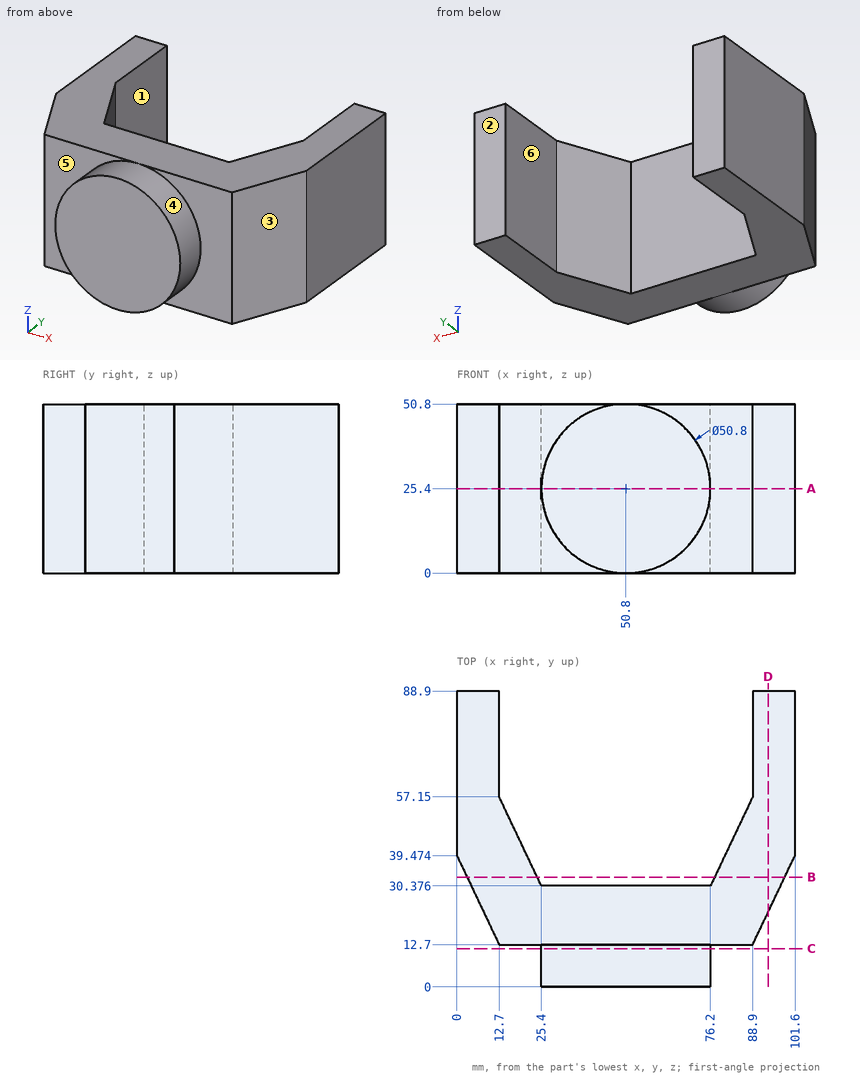
Geometry check sheet. Reference: drawing and pictorial views, mm from the part's lowest x, y, z. A direction names the side the tool comes from. Coordinates: 2 decimals unless noted, no trailing zeros. Write each loop counter-clockwise with the first axis right and the second up, starting at its lowest first coordinate (ties: lowest second). Pieces come first, ordered by that corner, then holes.
Item 1: Access from +Z, -Z, +X, -X, +Y, -Y to the whole of each face (thin tool, end or side, straight path). Record for the marked faces 4, 5 and 6.
Numbers:
face 4: -Y
face 5: -X, -Y
face 6: +Z, -Z, +Y
Item 2: Scan lines: probe 1 along X at (y, z) = (66, 39.5); probe 2 along X at (y, z) = (39.5, 39); probe 3 along Y at (x, z) = (58.5, 13). Record each from-to range of solid material in increasing order.
Numbers:
probe 1: x = 0 to 12.7, 88.9 to 101.6
probe 2: x = 0 to 21.07, 80.53 to 101.6
probe 3: y = 0 to 30.38
Item 3: Cross-section at D-D on x = 93.5. Record the boundary of the cut face in (y, z), then the cut area to 3 significant figures.
Numbers:
outline: (22.4, 0) - (88.9, 0) - (88.9, 50.8) - (22.4, 50.8) - close
area: 3,380 mm2
Item 4: Cross-section at C-C on y = 11.5. Record the boundary of the cut face in (x, z), then the cut area to 3 significant figures.
Numbers:
outline: circle Ø50.8 at (50.8, 25.4)
area: 2,030 mm2
Item 5: Cross-section at B-B on y = 33. Record the boundary of the cut face in (x, z).
Numbers:
outline: (3.07, 0) - (24.16, 0) - (24.16, 50.8) - (3.07, 50.8) - close; (77.44, 0) - (98.53, 0) - (98.53, 50.8) - (77.44, 50.8) - close
Item 6: Depth check by flat-ended pin: pin 1 Ø12 at (x, z) = (17.5, 24) entering from -Y; pin 2 Ø6 at (x, y) = (50.5, 24.5) entering from -Z; pin 3 Ø1.5 at (y, z) = (33, 5.5) entering from +X (3 decimals); pin 4 Ø8 at (y, z) = (16, 37.5) entering from -X. Enter the tip coordinate at first touch or a pass-through.
Numbers:
pin 1: stops at y = 12.7
pin 2: stops at z = 0
pin 3: stops at x = 98.885
pin 4: stops at x = 9.24
Item 7: Cross-section at A-A on z = 25.4. Record the boundary of the cut face in (x, y).
Numbers:
outline: (0, 39.47) - (12.7, 12.7) - (25.4, 12.7) - (25.4, 0) - (76.2, 0) - (76.2, 12.7) - (88.9, 12.7) - (101.6, 39.47) - (101.6, 88.9) - (88.9, 88.9) - (88.9, 57.15) - (76.2, 30.38) - (25.4, 30.38) - (12.7, 57.15) - (12.7, 88.9) - (0, 88.9) - close
Item 8: Mould release check, pull along X, two halves, no side actions. Record for the marked faces 1, 2 and 3: released by +X, released by -X, zero draft, split by the parting line, or undercut.
Numbers:
face 1: undercut
face 2: zero draft
face 3: released by +X
